```python
from build123d import *

# Parameters (mm, degrees)
SKETCH1_W            = 21.75
SKETCH1_H            = 29
BOSS_EXTRUDE1_DEPTH  = 16.6
SKETCH2_W            = 25.25
SKETCH2_H            = 31.5
BOSS_EXTRUDE2_DEPTH  = 2.1
SKETCH3_W            = 1.2
SKETCH3_H            = 29
BOSS_EXTRUDE3_DEPTH  = 13.85
BOSS_EXTRUDE4_START  = -3.65
BOSS_EXTRUDE4_DEPTH  = 18.3
SKETCH5_W            = 6
SKETCH5_H            = 0.8
BOSS_EXTRUDE6_DEPTH  = 11.35
CHAMFER2_SIZE        = 1.5
FILLET1_R            = 2
FILLET2_R            = 1.5
BOSS_EXTRUDE7_DEPTH  = 3.75
MIRROR2_COPY_1_DEPTH = 3.75


with BuildPart() as part:
    # Sketch1 → Boss-Extrude1 (new body)
    with BuildSketch(Plane(origin=(0, 0, 0), x_dir=(1, 0, 0), z_dir=(0, 1, 0))):
        Rectangle(SKETCH1_W, SKETCH1_H)
    extrude(amount=BOSS_EXTRUDE1_DEPTH)

    # Sketch2 → Boss-Extrude2 (add)
    with BuildSketch(Plane(origin=(0, 0, 0), x_dir=(1, 0, 0), z_dir=(0, 1, 0))):
        Rectangle(SKETCH2_W, SKETCH2_H)
    extrude(amount=BOSS_EXTRUDE2_DEPTH)

    # Sketch3 → Boss-Extrude3 (add)
    with BuildSketch(Plane(origin=(0, 16.6, 0), x_dir=(1, 0, 0), z_dir=(0, 1, 0))):
        Rectangle(SKETCH3_W, SKETCH3_H)
    extrude(amount=BOSS_EXTRUDE3_DEPTH)

    # Sketch4 → Boss-Extrude4 (add)
    with BuildSketch(Plane(origin=(12.625, 0, 0), x_dir=(0, 0, -1), z_dir=(1, 0, 0)).offset(BOSS_EXTRUDE4_START)):
        with BuildLine():
            Line((-12.25, 0), (-11.338972746, -3.4))
            ThreePointArc((-11.338972746, -3.4), (0, -1.6), (11.338972746, -3.4))
            Line((11.338972746, -3.4), (12.25, 0))
            Line((12.25, 0), (-12.25, 0))
        make_face()
    extrude(amount=-BOSS_EXTRUDE4_DEPTH)

    # Sketch5 → Boss-Extrude6 (add)
    with BuildSketch(Plane(origin=(0, 16.6, 0), x_dir=(1, 0, 0), z_dir=(0, 1, 0))):
        with Locations((5.4375, 9.8)):
            Rectangle(SKETCH5_W, SKETCH5_H)
        with Locations((5.4375, 0)):
            Rectangle(SKETCH5_W, SKETCH5_H)
        with Locations((5.4375, -9.8)):
            Rectangle(SKETCH5_W, SKETCH5_H)
        with Locations((-5.4375, -9.8)):
            Rectangle(SKETCH5_W, SKETCH5_H)
        with Locations((-5.4375, 0)):
            Rectangle(SKETCH5_W, SKETCH5_H)
        with Locations((-5.4375, 9.8)):
            Rectangle(SKETCH5_W, SKETCH5_H)
    extrude(amount=BOSS_EXTRUDE6_DEPTH)

    # Chamfer2
    chamfer2_edges = [part.edges().sort_by_distance(p)[0] for p in [
        (-2.4375, 27.95, 0),
        (-8.4375, 27.95, 0),
        (-2.4375, 27.95, -9.8),
        (-8.4375, 27.95, -9.8),
        (8.4375, 27.95, 0),
        (2.4375, 27.95, 0),
        (-2.4375, 27.95, 9.8),
        (-8.4375, 27.95, 9.8),
        (2.4375, 27.95, -9.8),
        (8.4375, 27.95, -9.8),
        (2.4375, 27.95, 9.8),
        (8.4375, 27.95, 9.8),
    ]]
    chamfer(chamfer2_edges, length=CHAMFER2_SIZE)

    # Fillet1
    fillet1_edges = [part.edges().sort_by_distance(p)[0] for p in [
        (12.625, 1.05, 15.75),
        (12.625, 1.05, -15.75),
        (-12.625, 1.05, -15.75),
        (-12.625, 1.05, 15.75),
    ]]
    fillet(fillet1_edges, radius=FILLET1_R)

    # Fillet2
    fillet2_edges = [part.edges().sort_by_distance(p)[0] for p in [
        (-0.175, -3.4, -11.338972746),
        (-0.175, -3.4, 11.338972746),
    ]]
    fillet(fillet2_edges, radius=FILLET2_R)

    # Sketch6 → Boss-Extrude7 (add)
    with BuildSketch(Plane.ZY.offset(10.875)):
        Polygon((-14.5, 16.6), (-16.8, 4.767525763), (-15.125, 2.1), (-14.5, 2.1), (-14.5, 2.609042619), (-15.954375498, 4.925212238), (-14.5, 12.407325549), align=None)
    boss_extrude7 = extrude(amount=-BOSS_EXTRUDE7_DEPTH)

    # Mirror1: Boss-Extrude7 across plane
    add(boss_extrude7.mirror(Plane(origin=(0, 0, 0), x_dir=(0, 0, 1), z_dir=(1, 0, 0))))

    # Mirror2: Boss-Extrude7 across plane
    add(boss_extrude7.mirror(Plane.XY))

    # Mirror2 copy 1 sketch → Mirror2 copy 1 (add)
    with BuildSketch(Plane(origin=(10.875, 0, 0), x_dir=(0, 0, -1), z_dir=(1, 0, 0))):
        Polygon((-14.5, 16.6), (-16.8, 4.767525763), (-15.125, 2.1), (-14.5, 2.1), (-14.5, 2.609042619), (-15.954375498, 4.925212238), (-14.5, 12.407325549), align=None)
    extrude(amount=-MIRROR2_COPY_1_DEPTH)


solid = part.part
```
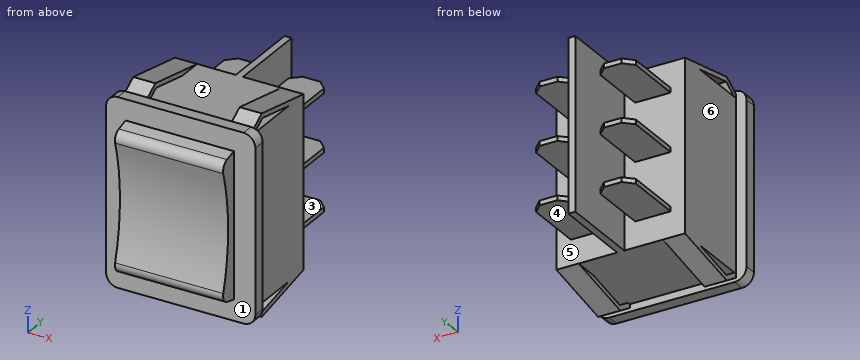
The model under review builds one solid part; all positions refer to its coordinate system, in mm. Face numbers are marked on the shaded views. A direction names the side the tool comes from. Round coordinates to 2 decimals unless told otherwise and drop trailing zeros. Loops run counter-clockwise (first coordinate to the right, second up) from the corner with the lowest first, then second, coordinate; pieces in that order, holes last. Notation, with made-up numbers: (25.5, 4) -> (35.5, 4) arc R29 ccw to (35.5, 40) -> close; hole circle Ø6 at (0, 63.5). An arc over 180 degrees is marked (long way). Answer in a Markdown table with one row per item.
1) Consider section A-A, the plane y = 24.5. Write out the cut boundary in (x, z).
Taken from the geometry:
| item | result |
|---|---|
| outline | (-8.44, -10.2) -> (-2.44, -10.2) -> (-2.44, -9.4) -> (-8.44, -9.4) -> close; (-8.44, -0.4) -> (-2.44, -0.4) -> (-2.44, 0.4) -> (-8.44, 0.4) -> close; (-8.44, 9.4) -> (-2.44, 9.4) -> (-2.44, 10.2) -> (-8.44, 10.2) -> close; (-0.6, -14.5) -> (0.6, -14.5) -> (0.6, 14.5) -> (-0.6, 14.5) -> close; (2.44, -10.2) -> (8.44, -10.2) -> (8.44, -9.4) -> (2.44, -9.4) -> close; (2.44, -0.4) -> (8.44, -0.4) -> (8.44, 0.4) -> (2.44, 0.4) -> close; (2.44, 9.4) -> (8.44, 9.4) -> (8.44, 10.2) -> (2.44, 10.2) -> close |
2) Draft analysis for pull direction Z (two halves, no side actions). For the marked faces 4, 5 and 6, state which applies: pulls with the +Z half, pulls with the -Z half, needs draft (parallel to the pull), parting line crosses it, or undercut.
Taken from the geometry:
| item | result |
|---|---|
| face 4 | pulls with the -Z half |
| face 5 | undercut |
| face 6 | needs draft |
3) Wall thickness on line 1 along Z through (x, y) = (7.5, 17.5); line 2 along Z through (x, y) = (2.5, 16.5); line 3 along X through (y, z) = (15.5, -5) (3 decimals): over which ranges is each line inside the solid? List them lowest first.
Taken from the geometry:
| item | result |
|---|---|
| line 1 | z = -10.2 to -9.4, -0.4 to 0.4, 9.4 to 10.2 |
| line 2 | z = -14.5 to 14.5 |
| line 3 | x = -10.875 to 10.875 |
4) For pin 1 Ø0.9 at (x, z) = (5.5, -10) entering from +Y; pin 2 Ø5 at (y, z) = (2.5, -10) entering from -X (3 decimals); pin 3 Ø1.5 at (x, z) = (-7.5, -3) entering from +Y; pin 4 Ø12 at (x, y) = (-8, 22.5) entering from +Z, all flat-tipped, find the tip position at first contact; note any pin that passes through.
Taken from the geometry:
| item | result |
|---|---|
| pin 1 | stops at y = 27.95 |
| pin 2 | stops at x = -12.625 |
| pin 3 | stops at y = 16.6 |
| pin 4 | stops at z = 14.52 |
5) Consider section C-C, the plane y = 8. Write out the cut boundary in (x, z) (3 decimals), plus the area to 3 significant figures.
Taken from the geometry:
| item | result |
|---|---|
| outline | (-10.875, -16.172) -> (-7.125, -16.172) -> (-7.125, -15.357) -> (-10.875, -15.357) -> close; (-10.875, -14.5) -> (10.875, -14.5) -> (10.875, 14.5) -> (-10.875, 14.5) -> close; (-10.875, 15.357) -> (-7.125, 15.357) -> (-7.125, 16.172) -> (-10.875, 16.172) -> close; (7.125, -16.172) -> (10.875, -16.172) -> (10.875, -15.357) -> (7.125, -15.357) -> close; (7.125, 15.357) -> (10.875, 15.357) -> (10.875, 16.172) -> (7.125, 16.172) -> close |
| area | 643 mm² |
6) Consider section B-B, the plane x = -5. Write out the cut boundary in (y, z).
Taken from the geometry:
| item | result |
|---|---|
| outline | (-2.96, -9.89) arc R1.5 ccw to (-1.9, -11.74) -> (0, -12.25) -> (0, -15.75) -> (2.1, -15.75) -> (2.1, -14.5) -> (16.6, -14.5) -> (16.6, -10.2) -> (27.95, -10.2) -> (27.95, -9.4) -> (16.6, -9.4) -> (16.6, -0.4) -> (27.95, -0.4) -> (27.95, 0.4) -> (16.6, 0.4) -> (16.6, 9.4) -> (27.95, 9.4) -> (27.95, 10.2) -> (16.6, 10.2) -> (16.6, 14.5) -> (2.1, 14.5) -> (2.1, 15.75) -> (0, 15.75) -> (0, 12.25) -> (-1.9, 11.74) arc R1.5 ccw to (-2.96, 9.89) arc R36.61 cw to start |
7) Consider section D-D, the plane z = 1.5. Write out the cut boundary in (x, y) (3 decimals).
Taken from the geometry:
| item | result |
|---|---|
| outline | (-12.625, 0) -> (-9.325, 0) -> (-9.325, -1.631) -> (8.975, -1.631) -> (8.975, 0) -> (12.625, 0) -> (12.625, 2.1) -> (10.875, 2.1) -> (10.875, 16.6) -> (0.6, 16.6) -> (0.6, 30.45) -> (-0.6, 30.45) -> (-0.6, 16.6) -> (-10.875, 16.6) -> (-10.875, 2.1) -> (-12.625, 2.1) -> close |
8) Tool access review of the marked faces 1, 2 and 3: name each direction out of +Z, -Z, +X, -X, +Y, -Y from which nothing blocks a thin tool from reaching the whole face with its end or side.
Taken from the geometry:
| item | result |
|---|---|
| face 1 | -Y |
| face 2 | none |
| face 3 | +X, +Y |
